```python
from build123d import *

# Parameters (mm, degrees)
F0_W     = 152.4
F0_H     = 76.2
F1_DEPTH = 2.9718
F2_R     = 25.4
F3_W     = 12.7
F3_H     = 2.9718
F3_W_2   = 6.35
F4_DEPTH = 25.4
F5_W     = 2.9718
F5_H     = 6.35
F6_DEPTH = 25.4


with BuildPart() as f1:
    # F0 (on Top) → F1 (new body)
    with BuildSketch(Plane.XY):
        Rectangle(F0_W, F0_H)
    extrude(amount=F1_DEPTH)

    # F2
    f2_edges = [f1.edges().sort_by_distance(p)[0] for p in [
        (-76.2, -38.1, 1.4859),
        (76.2, -38.1, 1.4859),
        (76.2, 38.1, 1.4859),
        (-76.2, 38.1, 1.4859),
    ]]
    fillet(f2_edges, radius=F2_R)

    # F3 (on face) → F4 (cut)
    with BuildSketch(Plane.XY.offset(2.9718)):
        Rectangle(F3_W, F3_H)
        with Locations((22.225, 0)):
            Rectangle(F3_W_2, F3_H)
        with Locations((-22.225, 0)):
            Rectangle(F3_W_2, F3_H)
    extrude(amount=-F4_DEPTH, mode=Mode.SUBTRACT)

    # F5 (on face) → F6 (cut)
    with BuildSketch(Plane.XY.offset(2.9718)):
        with Locations((23.9141, 12.7)):
            Rectangle(F5_W, F5_H)
        with Locations((23.9141, -12.7)):
            Rectangle(F5_W, F5_H)
        with Locations((-23.9141, 12.7)):
            Rectangle(F5_W, F5_H)
        with Locations((-23.9141, -12.7)):
            Rectangle(F5_W, F5_H)
    extrude(amount=-F6_DEPTH, mode=Mode.SUBTRACT)


solid = f1.part
```
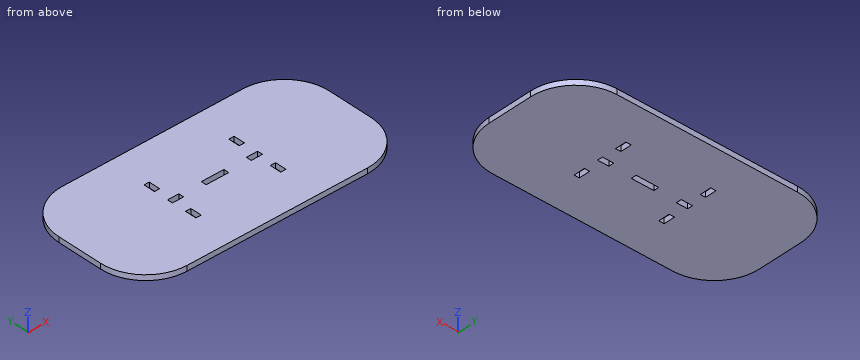
Could you check a few things on this model? Use its own coordinates, in mm. Give positions to 0.01 mm unless a question says otherwise; leave off trailing zeros. Loops run counter-clockwise (first coordinate to the right, second up) from the corner with the lowest first, then second, coordinate; pieces in that order, holes last. Notation, with made-up numbers: (50, -18.75) - (75, -18.75) arc R27 cw to (75, 20.25) - close; hole circle Ø4 at (-28, 55). An arc over 180 degrees is marked (long way). Answer in a Markdown table with one row per item. Add a question column.
Q1. If we section it at A-A (z = 2.5): State how many separate pieces and enclosed holes the cut face has, plus the area to 3 significant figures.
Q2. If we section it at C-C (x = -65.5): List the corners of the cut face in (y, z) for me, plus the area to 3 significant figures.
Q3. Please list where these lines run through material, in increasing order: L1, parallel to X at y = -10.5, z = 0.6; L2, parallel to Y at x = -25, z = 2.2 (3 decimals); L3, parallel to X at y = 15.5, z = 1.75. Write a range as from..to.
Q4. For pin 1 (1.5 mm diameter, centred on y = 13, z = 1.5, fed in from -X), with a flat end and sliding along its axis, tell me the tip position at first contact or that it passes through.
Q5. If we section it at B-B (y = -29.5): List the corners of the cut face in (x, z) for me, plus the area to 3 significant figures.
The answers:
| question | item | result |
|---|---|---|
| 1 | separate pieces | 1 |
| 1 | enclosed holes | 7 |
| 1 | area | 10,900 mm^2 |
| 2 | outline | (-33.41, 0) - (33.41, 0) - (33.41, 2.97) - (-33.41, 2.97) - close |
| 2 | area | 199 mm^2 |
| 3 | L1 | x = -76.2..-25.4, -22.43..22.43, 25.4..76.2 |
| 3 | L2 | y = -38.1..-15.875, -9.525..-1.486, 1.486..9.525, 15.875..38.1 |
| 3 | L3 | x = -76.05..-25.4, -22.43..22.43, 25.4..76.05 |
| 4 | pin 1 | stops at x = -76.2 |
| 5 | outline | (-69.85, 0) - (69.85, 0) - (69.85, 2.97) - (-69.85, 2.97) - close |
| 5 | area | 415 mm^2 |
